from build123d import *

# Parameters (mm, degrees)
SKETCH073_W = 22.4
SKETCH073_H = 34.4
SKETCH074_W = 22.4
SKETCH074_H = 23.4
SKETCH075_W = 22.4
SKETCH075_H = 23.4
SKETCH072_R = 17
SKETCH076_W = 22.4
SKETCH076_H = 34.4


with BuildPart() as loft008:
    # Sketch073 → Loft008 section 0
    with BuildSketch(Plane(origin=(24, 0, 19.5), x_dir=(0, 1, 0), z_dir=(1, 0, 0))):
        with Locations((0, 6.2)):
            Rectangle(SKETCH073_W, SKETCH073_H)
    # Sketch074 → Loft008 section 1
    with BuildSketch(Plane(origin=(12, 0, 19.5), x_dir=(0, 1, 0), z_dir=(1, 0, 0))):
        with Locations((0, 13.2)):
            Rectangle(SKETCH074_W, SKETCH074_H)
    # Sketch075 → Loft008 section 2
    with BuildSketch(Plane(origin=(-2, 0, 19.5), x_dir=(0, 1, 0), z_dir=(1, 0, 0))):
        with Locations((0, 13.2)):
            Rectangle(SKETCH075_W, SKETCH075_H)
    loft(ruled=True)


with BuildPart() as fusion005:
    # Sketch072 → Loft007 section 0
    with BuildSketch(Plane(origin=(30, 0, 19.5), x_dir=(0, 1, 0), z_dir=(1, 0, 0))):
        with Locations((0, 6.4)):
            Circle(SKETCH072_R)
    # Sketch076 → Loft007 section 1
    with BuildSketch(Plane(origin=(24, 0, 19.5), x_dir=(0, 1, 0), z_dir=(1, 0, 0))):
        with Locations((0, 6.2)):
            Rectangle(SKETCH076_W, SKETCH076_H)
    loft()

    # Fusion005: union Loft008
    add(loft008.part)


solid = fusion005.part
Geometry check sheet. Reference: the model listing, model coordinates, mm. A direction names the side the tool comes from. Round coordinates to 2 decimals unless told otherwise and drop trailing zeros. Loops run counter-clockwise (first coordinate to the right, second up) from the corner with the lowest first, then second, coordinate; pieces in that order, holes last. Notation, with made-up numbers: (-6.5, 76.25) - (34.5, 76.25) arc R20 ccw to (34.5, 102.25) - close; hole circle Ø3 at (43.5, 85.5). An arc over 180 degrees is marked (long way). One line per question, with ' | ' between items. Start each with the question number.
1. Tool access check on faces 1 (the face through (11, 11.2, 30)), 2 (the face through (5, 0, 21)), 3 (the face through (5, 0, 44.4)), 4 (the face through (11, -11.2, 31)). Record the directions out of +Z, -Z, +X, -X, +Y, -Y that give a thin tool (end or side, any length) a straight path to the whole face; none if there is none.
2. Cross-section at A-A on x = 9. Record the cut outline in (y, z), then the cut area to 3 significant figures.
3. Depth check by flat-ended pin: pin 1 (3 mm diameter, centred on x = 14.5, z = 32.5, fed in from -Y); pin 2 (8 mm diameter, centred on x = 15, y = -10, fed in from -Z); pin 3 (10 mm diameter, centred on x = 19.5, z = 38, fed in from +Y). Enter the tip coordinate at first touch or a pass-through.
4. Cross-section at B-B on x = 23. Record the cut outline in (y, z) (3 decimals).
5. Scan lines: line 1 (Y direction, x = 8.5, z = 21.5); line 2 (Z direction, x = 8, y = 7); line 3 (X direction, y = -3, z = 10). Record each from-to range of solid material in increasing order. Write a range as [from, to].
Taken from the geometry:
1) face 1: +Z, -Z, -X, +Y | face 2: -Z, -X, +Y, -Y | face 3: +Z, +X, -X, +Y, -Y | face 4: +Z, -Z, -X, -Y
2) outline: (-11.2, 21) - (11.2, 21) - (11.2, 44.4) - (-11.2, 44.4) - close | area: 524 mm²
3) pin 1: y = -11.2 | pin 2: z = 13.71 | pin 3: y = 11.36
4) outline: (-11.2, 9.542) - (11.2, 9.542) - (11.2, 43.025) - (-11.2, 43.025) - close
5) line 1: [-11.2, 11.2] | line 2: [21, 44.4] | line 3: [22.56, 30]
